```python
from build123d import *

# Parameters (mm, degrees)
CROQUIS1_R     = 11
EXTRUIR1_DEPTH = 0.7
CROQUIS2_R     = 9.775
CROQUIS2_R_2   = 9.075
CROQUIS2_R_3   = 7.85
CROQUIS2_R_4   = 7.15
CROQUIS2_R_5   = 5.925
CROQUIS2_R_6   = 5.225
EXTRUIR2_DEPTH = 1.6
CROQUIS3_R     = 4.7
EXTRUIR3_DEPTH = 1.6


with BuildPart() as part:
    # Croquis1 → Extruir1 (new body)
    with BuildSketch(Plane(origin=(0, 0, 0), x_dir=(1, 0, 0), z_dir=(0, 1, 0))):
        with Locations(Location((0, 0, 0), (0, 0, 270))):
            Circle(CROQUIS1_R)
    extrude(amount=EXTRUIR1_DEPTH)

    # Croquis2 → Extruir2 (add)
    # profile 1 of 3: a face of its own
    with BuildSketch(Plane(origin=(0, 0.7, 0), x_dir=(1, 0, 0), z_dir=(0, 1, 0))):
        with Locations(Location((0, 0, 0), (0, 0, 270))):
            Circle(CROQUIS2_R)
        with Locations(Location((0, 0, 0), (0, 0, 270))):
            Circle(CROQUIS2_R_2, mode=Mode.SUBTRACT)
    # profile 2 of 3: a face of its own
    with BuildSketch(Plane(origin=(0, 0.7, 0), x_dir=(1, 0, 0), z_dir=(0, 1, 0))):
        with Locations(Location((0, 0, 0), (0, 0, 270))):
            Circle(CROQUIS2_R_3)
        with Locations(Location((0, 0, 0), (0, 0, 270))):
            Circle(CROQUIS2_R_4, mode=Mode.SUBTRACT)
    # profile 3 of 3: a face of its own
    with BuildSketch(Plane(origin=(0, 0.7, 0), x_dir=(1, 0, 0), z_dir=(0, 1, 0))):
        with Locations(Location((0, 0, 0), (0, 0, 270))):
            Circle(CROQUIS2_R_5)
        with Locations(Location((0, 0, 0), (0, 0, 270))):
            Circle(CROQUIS2_R_6, mode=Mode.SUBTRACT)
    extrude(amount=EXTRUIR2_DEPTH)

    # Croquis3 → Extruir3 (cut)
    with BuildSketch(Plane(origin=(0, 0.7, 0), x_dir=(1, 0, 0), z_dir=(0, 1, 0))):
        with Locations(Location((0, 0, 0), (0, 0, 270))):
            Circle(CROQUIS3_R)
    extrude(amount=-EXTRUIR3_DEPTH, mode=Mode.SUBTRACT)


solid = part.part
```
Read the model definition and answer for the solid it produces. Units are mm, in the model's axes. A direction names the side the tool comes from. Round coordinates to 2 decimals unless told otherwise and drop trailing zeros. Write each loop counter-clockwise with the first axis right and the second up, starting at its lowest first coordinate (ties: lowest second). Pieces come first, ordered by that corner, then holes. Notation, with made-up numbers: (-37, 13) - (-5, 13) arc R13 ccw to (-5, 27) - close; hole circle Ø1 at (6.25, -34). An arc over 180 degrees is marked (long way). One line per item, written item: value.
Q1. Which of the six approach directions +Z, -Z, +X, -X, +Y, -Y give full straight-line access (tool end or side, diameter ignored) to faces 4 (the cylindrical face through (1.412, 0.355, 4.483)), 5 (the flat face through (6, 0.7, 1))?
The answers:
face 4: +Y, -Y
face 5: +Y
Q2. Find section A-A (y = 0.95). Determine the outline of the cut face in (x, z) (3 decimals), and give its area (3 significant figures).
The answers:
outline: circle Ø19.55 at (0, 0); circle Ø15.7 at (0, 0); circle Ø11.85 at (0, 0); hole circle Ø18.15 at (0, 0); hole circle Ø14.3 at (0, 0); hole circle Ø10.45 at (0, 0)
area: 99.0 mm2
Q3. For a pull along X with two mould halves and no side action, classify faces 1 (the flat face through (-9, 2.3, 3)), 2 (the cylindrical face through (2.936, 1.489, 9.324)), 3 (the flat face through (7, 0.7, -4)) as pulls with the +X half, pulls with the -X half, needs draft (parallel to the pull), parting line crosses it, or undercut.
The answers:
face 1: needs draft
face 2: parting line crosses it
face 3: undercut
Q4. Straight lines are drawn through the part: line 1 (X direction, y = 1.95, z = 0) (3 decimals); line 2 (X direction, y = 1.75, z = -3.5); line 3 (Z direction, x = 2.75, y = 1.35). For each, find the intervals that lie inside material, in ascending order. Write a range as from..to.
The answers:
line 1: x = -9.775..-9.075, -7.85..-7.15, -5.925..-5.225, 5.225..5.925, 7.15..7.85, 9.075..9.775
line 2: x = -9.13..-8.37, -7.03..-6.23, -4.78..-3.88, 3.88..4.78, 6.23..7.03, 8.37..9.13
line 3: z = -9.38..-8.65, -7.35..-6.6, -5.25..-4.44, 4.44..5.25, 6.6..7.35, 8.65..9.38
Q5. Each of these flat-tipped pins is pushed along its axis until it touches: P1, Ø8.5, axis at x = -2, z = -1.5, coming from the +Y side; P2, Ø1, axis at x = 1, y = 1.5, coming from the +Z side. Where does it stop, or does it pass through?
The answers:
P1: stops at y = 2.3
P2: stops at z = 9.76
